```python
from build123d import *

# Parameters (mm, degrees)
BOSS_EXTRUDE1_DEPTH  = 20
CHAMFER1_SIZE        = 10
M8_CLEARANCE_HOLE1_D = 8.4
SKETCH13_W           = 20.4
SKETCH13_H           = 20.4
CUT_EXTRUDE1_DEPTH   = 10


# Read off the part's stored shape, not the designer's step: Revolve1
with BuildPart() as part:
    # Sketch1 → Boss-Extrude1 (new body)
    with BuildSketch(Plane(origin=(0, 0, 0), x_dir=(1, 0, 0), z_dir=(0, 1, 0))):
        with BuildLine():
            Line((25, 250), (25, -250))
            ThreePointArc((25, -250), (0, -275), (-25, -250))
            Line((-25, -250), (-25, 250))
            ThreePointArc((-25, 250), (0, 275), (25, 250))
        make_face()
        with BuildLine():
            Line((-250, 25), (250, 25))
            ThreePointArc((250, 25), (275, 0), (250, -25))
            Line((250, -25), (-250, -25))
            ThreePointArc((-250, -25), (-275, 0), (-250, 25))
        make_face()
    extrude(amount=BOSS_EXTRUDE1_DEPTH)

    # Chamfer1
    chamfer1_edges = [part.edges().sort_by_distance(p)[0] for p in [
        (275, 20, 0),
        (137.5, 20, 25),
        (137.5, 20, -25),
        (-137.5, 20, -25),
        (25, 10, -25),
        (-25, 10, -25),
        (25, 10, 25),
        (-25, 10, 25),
        (25, 20, -137.5),
        (25, 20, 137.5),
        (0, 20, 275),
        (-25, 20, -137.5),
        (-25, 20, 137.5),
        (0, 20, -275),
        (-275, 20, 0),
        (-137.5, 20, 25),
    ]]
    chamfer(chamfer1_edges, length=CHAMFER1_SIZE)

    # M8 Clearance Hole1 (through all)
    with Locations(Plane(origin=(0, 20, 0), x_dir=(1, 0, 0), z_dir=(0, 1, 0))):
        with Locations((-250, 0), (0, 250), (250, 0), (0, -250)):
            Hole(M8_CLEARANCE_HOLE1_D / 2)

    # Sketch13 → Cut-Extrude1 (cut)
    with BuildSketch(Plane(origin=(0, 20, 0), x_dir=(1, 0, 0), z_dir=(0, 1, 0))):
        Rectangle(SKETCH13_W, SKETCH13_H)
    extrude(amount=-CUT_EXTRUDE1_DEPTH, mode=Mode.SUBTRACT)

    # Revolve1 outline → Revolve1 (revolve)
    with BuildSketch(Plane.XY):
        with BuildLine():
            ThreePointArc((26.958266811, 20), (22.909428257, 21.591165693), (21, 25.5))
            ThreePointArc((21, 25.5), (19.090571743, 21.591165693), (15.041733189, 20))
            Line((15.041733189, 20), (26.958266811, 20))
        make_face()
    revolve(axis=Axis((0, 0, 0), (0, 1, 0)))


solid = part.part
```
The model under review builds one solid part; all positions refer to its coordinate system, in mm. A direction names the side the tool comes from. Round coordinates to 2 decimals unless told otherwise and drop trailing zeros. Loops run counter-clockwise (first coordinate to the right, second up) from the corner with the lowest first, then second, coordinate; pieces in that order, holes last. Notation, with made-up numbers: (73.25, -13.5) -> (110.25, -13.5) arc R19 ccw to (110.25, 19.5) -> close; hole circle Ø2 at (42, 59.25). An arc over 180 degrees is marked (long way). Answer as a JSON object with one key per item and string values. Group by question number.
1) We need section A-A on y = 14.25. Write out the cut boundary in (x, z).
2) For line 1 (Z direction, x = 0, y = 4.25); line 2 (Z direction, x = 0, y = 13); line 3 (Y direction, x = 5.5, z = -143.5), list the stretches that pass through material, from the lowest coordinate up. Write a range as [from, to].
3) For faces 1 (the face through (0.55, 4.93, 274.994)), 2 (the face through (21, 20, -21)), list the 3-axis set-ups (+Z, -Z, +X, -X, +Y, -Y) from which the entire face can be reached by the end or side of a thin tool; tool diameter is ignored.
4) For pin 1 Ø8 at (y, z) = (5, -183.5) entering from -X; pin 2 Ø5 at (x, y) = (157, 6.5) entering from -Z; pin 3 Ø11 at (x, y) = (-2.5, 14) entering from +Z, all flat-tipped, find the tip position at first contact; note any pin that passes through.
5) We need section B-B on x = -162.5. Write out the cut boundary in (y, z).
6) Mouldability with a two-part tool opening along Z and no side actions: class faces 3 (the face through (0, 10, 0)), 4 (the face through (-27, 16, 27)), 5 (the face through (27, 16, -27)), 6 (the face through (267, 18, 0)) as released by +Z, released by -Z, zero draft, split by the parting line, or undercut.
7) We need section C-C on z = 90.5. Write out the cut boundary in (x, y).
Result set:
{
 "1": {"outline": "(-250, -20.75) -> (-35, -20.75) -> (-20.75, -35) -> (-20.75, -250) arc R20.75 ccw to (20.75, -250) -> (20.75, -35) -> (35, -20.75) -> (250, -20.75) arc R20.75 ccw to (250, 20.75) -> (35, 20.75) -> (20.75, 35) -> (20.75, 250) arc R20.75 ccw to (-20.75, 250) -> (-20.75, 35) -> (-35, 20.75) -> (-250, 20.75) arc R20.75 ccw to start; hole circle Ø8.4 at (-250, 0); hole (-10.2, -10.2) -> (10.2, -10.2) -> (10.2, 10.2) -> (-10.2, 10.2) -> close; hole circle Ø8.4 at (0, -250); hole circle Ø8.4 at (0, 250); hole circle Ø8.4 at (250, 0)"},
 "2": {"line 1": "[-275, -254.2], [-245.8, 245.8], [254.2, 275]", "line 2": "[-272, -254.2], [-245.8, -10.2], [10.2, 245.8], [254.2, 272]", "line 3": "[0, 20]"},
 "3": {"face 1": "+Z, +Y, -Y", "face 2": "+Y"},
 "4": {"pin 1": "x = -25", "pin 2": "z = -25", "pin 3": "z = 275"},
 "5": {"outline": "(0, -25) -> (10, -25) -> (20, -15) -> (20, 15) -> (10, 25) -> (0, 25) -> close"},
 "6": {"face 3": "undercut", "face 4": "released by +Z", "face 5": "released by -Z", "face 6": "split by the parting line"},
 "7": {"outline": "(-25, 0) -> (25, 0) -> (25, 10) -> (15, 20) -> (-15, 20) -> (-25, 10) -> close"}
}
